```python
from build123d import *

# Parameters (mm, degrees)
EXTRUDE_562_DEPTH    = 11.5
EXTRUDE_7_DEPTH      = 79
EXTRUDE_7_DEPTH_BACK = 11.5
SKETCH_2_W           = 1329
SKETCH_2_H           = 11.5
EXTRUDE_9_DEPTH      = 67.5
EXTRUDE_9_DEPTH_BACK = 11.5
SKETCH_3_W           = 1760
SKETCH_3_H           = 11.5
SKETCH_4_W           = 140
SKETCH_4_H           = 50
EXTRUDE_10_DEPTH     = 11.5


with BuildPart() as part:
    # 草图1 → Extrude 562 (new body)
    with BuildSketch(Plane.XY):
        Polygon((-744.5, 139.25), (-664.5, 59.25), (664.5, 59.25), (744.5, 139.25), (824.5, 139.25), (824.5, -139.25), (-824.5, -139.25), (-824.5, 139.25), align=None)
    extrude(amount=EXTRUDE_562_DEPTH)

    # 草图2 → 凸台-拉伸7 (add, two sides: drawn at the far end of the back side and taken through both)
    with BuildSketch(Plane.XY.offset(11.5).offset(-EXTRUDE_7_DEPTH_BACK)):
        with Locations((0, 65)):
            Rectangle(SKETCH_2_W, SKETCH_2_H)
    extrude(amount=EXTRUDE_7_DEPTH + EXTRUDE_7_DEPTH_BACK)

    # 草图3 → 凸台-拉伸9 (add, two sides: drawn at the far end of the back side and taken through both)
    with BuildSketch(Plane.XY.offset(11.5).offset(-EXTRUDE_9_DEPTH_BACK)):
        with Locations((0, -145)):
            Rectangle(SKETCH_3_W, SKETCH_3_H)
    extrude(amount=EXTRUDE_9_DEPTH + EXTRUDE_9_DEPTH_BACK)

    # 草图4 → 凸台-拉伸10 (add)
    with BuildSketch(Plane(origin=(0, -139.25, 0), x_dir=(-1, 0, 0), z_dir=(0, 1, 0))):
        with Locations((-790, 48)):
            Rectangle(SKETCH_4_W, SKETCH_4_H)
        with Locations((790, 48)):
            Rectangle(SKETCH_4_W, SKETCH_4_H)
    extrude(amount=EXTRUDE_10_DEPTH)


solid = part.part
```
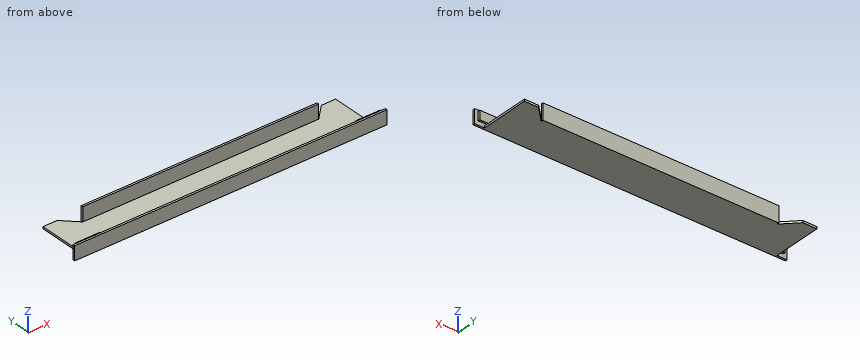
Input: part model. Units: mm. Frame: model coordinates. Coordinates: 2 decimals unless noted, no trailing zeros. Loops run counter-clockwise (first coordinate to the right, second up) from the corner with the lowest first, then second, coordinate; pieces in that order, holes last. Notation, with made-up numbers: M 32.25,9 L 74.25,9 A19 ccw 74.25,24 Z; hole C 36.5,-10 d11. An arc over 180 degrees is marked long. Answer in a Markdown table with one row per item.
1. Section A-A, the plane z = 41.5. Output: boundary loops of the cut face in (x, y), then the cut area to 3 significant figures.
Response:
| item | result |
|---|---|
| outline | M -880,-150.75 L 880,-150.75 L 880,-139.25 L 860,-139.25 L 860,-127.75 L 720,-127.75 L 720,-139.25 L -720,-139.25 L -720,-127.75 L -860,-127.75 L -860,-139.25 L -880,-139.25 Z; M -664.5,59.25 L 664.5,59.25 L 664.5,70.75 L -664.5,70.75 Z |
| area | 38,700 mm2 |
2. Section C-C, the plane y = -73.5. Output: boundary loops of the cut face in (x, z), then the cut area to 3 significant figures.
Response:
| item | result |
|---|---|
| outline | M -824.5,0 L 824.5,0 L 824.5,11.5 L -824.5,11.5 Z |
| area | 19,000 mm2 |
3. First-contact query: pin 1 (12.5 mm diameter, centred on y = 67.5, z = 44, fed in from -X); pin 2 (6 mm diameter, centred on x = 189.5, y = -147, fed in from +Z); pin 3 (3.5 mm diameter, centred on x = -806, y = -132.5, fed in from +Z). Flat tips, straight axial feed; report the tip coordinate or a pass-through.
Response:
| item | result |
|---|---|
| pin 1 | stops at x = -664.5 |
| pin 2 | stops at z = 79 |
| pin 3 | stops at z = 73 |
4. Section B-B, the plane x = -467.5. Output: boundary loops of the cut face in (y, z).
Response:
| item | result |
|---|---|
| outline | M -150.75,0 L 70.75,0 L 70.75,90.5 L 59.25,90.5 L 59.25,11.5 L -139.25,11.5 L -139.25,79 L -150.75,79 Z |
5. Material intervals for line 1 (Y direction, x = -53.5, z = 22); line 2 (Z direction, x = 138.5, y = -59); line 3 (X direction, y = -129, z = 57), sorted ascending.
Response:
| item | result |
|---|---|
| line 1 | y = -150.75 to -139.25, 59.25 to 70.75 |
| line 2 | z = 0 to 11.5 |
| line 3 | x = -860 to -720, 720 to 860 |
6. Section D-D, the plane x = 774.5. Output: boundary loops of the cut face in (y, z), then the cut area to 3 significant figures.
Response:
| item | result |
|---|---|
| outline | M -150.75,0 L 139.25,0 L 139.25,11.5 L -139.25,11.5 L -139.25,23 L -127.75,23 L -127.75,73 L -139.25,73 L -139.25,79 L -150.75,79 Z |
| area | 4,690 mm2 |
